Can you work these out from the model? Positions are in its coordinate system, mm. Face numbers are marked on the shaded views. A direction names the side the tool comes from. Coordinates: 2 decimals unless noted, no trailing zeros. Loops run counter-clockwise (first coordinate to the right, second up) from the corner with the lowest first, then second, coordinate; pieces in that order, holes last. Notation, with made-up numbers: M -17.75,-18 L 0.25,-18 A19 ccw 0.25,-13 Z; hole C -17.5,25.5 d11. An arc over 180 degrees is marked long. Return JSON: item names as keys, results as strings. Group by question number.
```python
from build123d import *

# Parameters (mm, degrees)
BASE_EXTRUDE_DEPTH     = 25
M10_GEVINDHULLER_D     = 8.5
M10_GEVINDHULLER_DEPTH = 19
M10_GEVINDHULLER_TIP   = 2.553657631


with BuildPart() as part:
    # Sketch1 → Base-Extrude (new body)
    with BuildSketch(Plane.XY):
        with BuildLine():
            Line((-11.04340479, 5.149624226), (-103.452365235, 48.240630163))
            ThreePointArc((-103.452365235, 48.240630163), (-111.867828916, 55.620793737), (-115, 66.366785904))
            Line((-115, 66.366785904), (-115, 82))
            ThreePointArc((-115, 82), (-116.97393957, 84.819077862), (-120.298133329, 83.928362829))
            Line((-120.298133329, 83.928362829), (-122.298133329, 81.544855644))
            ThreePointArc((-122.298133329, 81.544855644), (-122.819077862, 80.642553245), (-123, 79.616492815))
            Line((-123, 79.616492815), (-123, 59.102819238))
            ThreePointArc((-123, 59.102819238), (-121.707567052, 50.39215945), (-117.941627071, 42.432029243))
            Line((-117.941627071, 42.432029243), (-99.553694394, 14.921337813))
            ThreePointArc((-99.553694394, 14.921337813), (-97.750312833, 12.887914315), (-95.466001321, 11.41518994))
            Line((-95.466001321, 11.41518994), (-34.123617057, -17.189233611))
            ThreePointArc((-34.123617057, -17.189233611), (-27.938257623, -19.288880214), (-21.445069205, -20))
            Line((-21.445069205, -20), (21.445069205, -20))
            ThreePointArc((21.445069205, -20), (27.938257623, -19.288880214), (34.123617057, -17.189233611))
            Line((34.123617057, -17.189233611), (95.466001321, 11.41518994))
            ThreePointArc((95.466001321, 11.41518994), (97.750312833, 12.887914315), (99.553694394, 14.921337813))
            Line((99.553694394, 14.921337813), (117.941627071, 42.432029243))
            ThreePointArc((117.941627071, 42.432029243), (121.707567052, 50.39215945), (123, 59.102819238))
            Line((123, 59.102819238), (123, 79.616492815))
            ThreePointArc((123, 79.616492815), (122.819077862, 80.642553245), (122.298133329, 81.544855644))
            Line((122.298133329, 81.544855644), (120.298133329, 83.928362829))
            ThreePointArc((120.298133329, 83.928362829), (116.97393957, 84.819077862), (115, 82))
            Line((115, 82), (115, 66.366785904))
            ThreePointArc((115, 66.366785904), (111.867828916, 55.620793737), (103.452365235, 48.240630163))
            Line((103.452365235, 48.240630163), (11.04340479, 5.149624226))
            ThreePointArc((11.04340479, 5.149624226), (10.379689702, 4.726139346), (9.84900766, 4.144560692))
            ThreePointArc((9.84900766, 4.144560692), (0, -1), (-9.84900766, 4.144560692))
            ThreePointArc((-9.84900766, 4.144560692), (-10.379689702, 4.726139346), (-11.04340479, 5.149624226))
        make_face()
    extrude(amount=BASE_EXTRUDE_DEPTH)

    # M10 gevindhuller
    with Locations(Plane(origin=(0, 0, 0), x_dir=(-1, 0, 0), z_dir=(0, 0, -1))):
        with Locations((-40, 3.205015461), (-62.657694676, 13.770472004), (-85.315389352, 24.335928548), (85.315389352, 24.335928548), (62.657694676, 13.770472004), (40, 3.205015461)):
            Hole(M10_GEVINDHULLER_D / 2, depth=M10_GEVINDHULLER_DEPTH)
            with Locations((0, 0, -(M10_GEVINDHULLER_DEPTH + M10_GEVINDHULLER_TIP / 2))):  # 118° drill point
                Cone(0, M10_GEVINDHULLER_D / 2, M10_GEVINDHULLER_TIP, mode=Mode.SUBTRACT)


solid = part.part
```
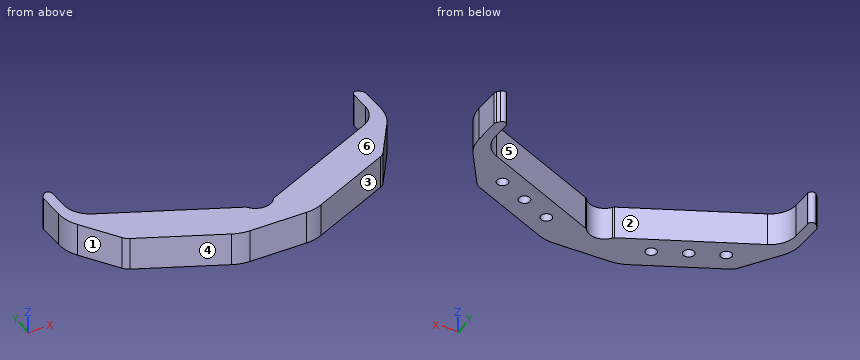
1) For pin 1 (5 mm diameter, centred on y = -5, z = 6.5, fed in from +X); pin 2 (2 mm diameter, centred on x = 64, z = 18.5, fed in from -Y); pin 3 (3 mm diameter, centred on y = -5.5, z = 5.5, fed in from +X), each with a flat end and sliding along its axis, tell me the tip position at first contact or that it passes through.
2) Suppose I cut it at C-C, the plane x = -107. List the corners of the cut face in (y, z) for me, then the cut area to 3 significant figures.
3) If we mould it in two halves opening along X, with no side actions, what happens to the marked faces 3, 4, 5 and 6? For each: +X half, -X half, draft (parallel to the pull), parting line (faces both ways), or undercut.
4) Suppose I cut it at D-D, the plane x = -53. List the corners of the cut face in (y, z) for me.
5) Suppose I cut it at A-A, the plane y = 75. List the corners of the cut face in (x, z) for me, then the cut area to 3 significant figures.
6) If I drill on line 1 (X direction, y = 73.5, z = 1.25); line 2 (X direction, y = 30, z = 6.5); line 3 (X direction, y = 11.5, z = 4) (3 decimals), over which ranges is the centre line in solid material (lowest first)? Write a range as from..to.
7) Suppose I cut it at B-B, the plane z = 9. Give the number of separate pieces and of enclosed holes in the cut face, then the cut area to 3 significant figures.
8) For the marked faces 1 and 2, which set-ups out of +Z, -Z, +X, -X, +Y, -Y let a thin tool reach every point of the face, with its end or its side?
Returned:
{
 "1": {"pin 1": "stops at x = 65.62", "pin 2": "stops at y = -3.72", "pin 3": "stops at x = 62.41"},
 "2": {"outline": "M 26.06,0 L 50.37,0 L 50.37,25 L 26.06,25 Z", "area": "608 mm²"},
 "3": {"face 3": "+X half", "face 4": "-X half", "face 5": "undercut", "face 6": "draft"},
 "4": {"outline": "M -8.39,0 L 24.71,0 L 24.71,25 L -8.39,25 Z"},
 "5": {"outline": "M -123,0 L -115,0 L -115,25 L -123,25 Z; M 115,0 L 123,0 L 123,25 L 115,25 Z", "area": "400 mm²"},
 "6": {"line 1": "x = -123..-115, 115..123", "line 2": "x = -109.63..-64.34, 64.34..109.63", "line 3": "x = -95.643..-66.25, -59.065..-24.662, 24.662..59.065, 66.25..95.643"},
 "7": {"separate pieces": "1", "enclosed holes": "6", "area": "7,240 mm²"},
 "8": {"face 1": "+Z, -Z, -X, -Y", "face 2": "+Z, -Z, +Y"}
}
